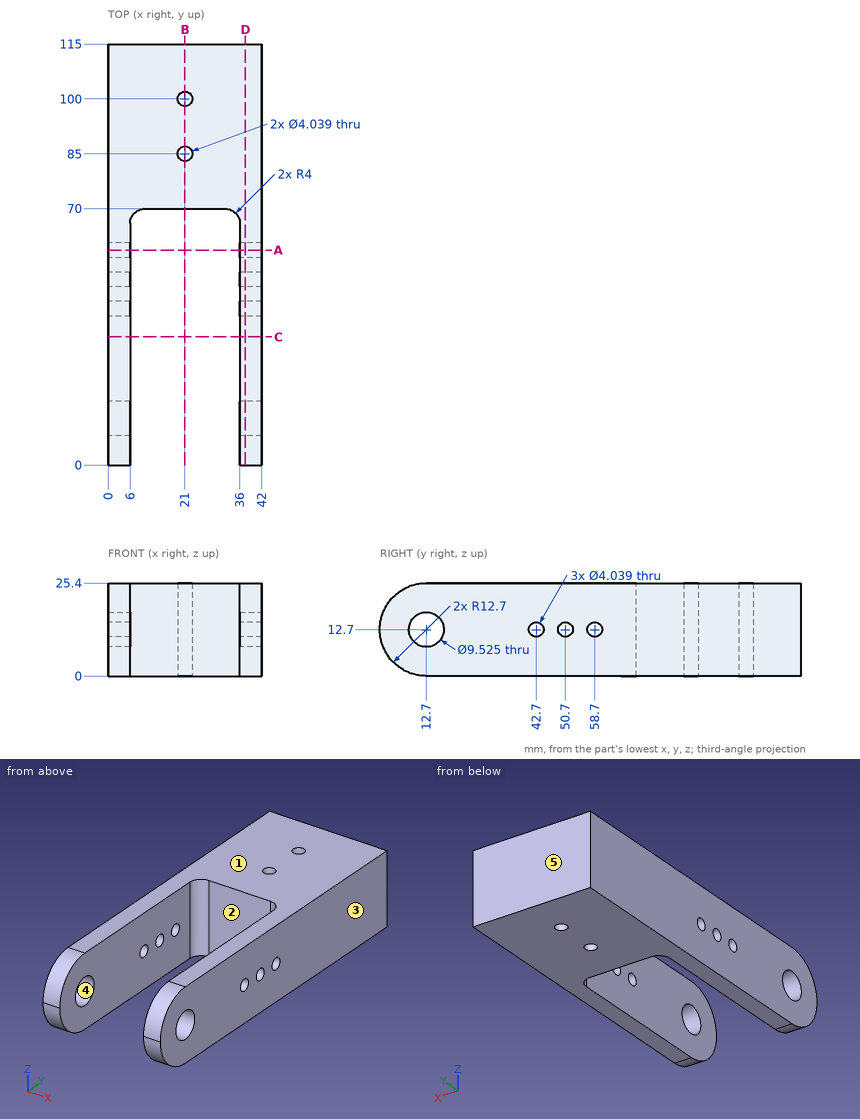
Could you check a few things on this drawing? It's one solid part, dimensions in mm from its lowest x, y, z. A direction names the side the tool comes from. Round coordinates to 2 decimals unless told otherwise and drop trailing zeros. Write each loop counter-clockwise with the first axis right and the second up, starting at its lowest first coordinate (ties: lowest second). Pieces come first, ordered by that corner, then holes.
Q1. If we section it at C-C on y = 35: Write out the boundary of the cut face in (x, z), plus the area to 3 significant figures.
Q2. Please list where these lines run through material, in increasing order: probe 1 along Y at (x, z) = (3.65, 12.7); probe 2 along Y at (x, z) = (21, 15.75); probe 3 along X at (y, z) = (35.5, 15.5).
Q3. If we section it at B-B on x = 21: Write out the boundary of the cut face in (y, z), plus the area to 3 significant figures.
Q4. If we section it at A-A on y = 58.7: Write out the boundary of the cut face in (x, z), plus the area to 3 significant figures.
Q5. If we mould it in two halves opening along Y, with no side actions, what happens to the marked faces 3, 4 and 5? For each: +Y half, -Y half, draft (parallel to the pull), parting line (faces both ways), or undercut.
Q6. Will these pins go through, and if not, where does the flat tip stop? P1, Ø4, axis at x = 9, z = 5, coming from the -Y side (1 decimal); P2, Ø11, axis at x = 16.5, z = 7.5, coming from the -Y side.
Q7. If we section it at D-D on x = 37.5: Give the number of separate pieces and of enclosed holes in the cut face, plus the area to 3 significant figures.
Q8. Which directions (+Z, -Z, +X, -X, +Y, -Y) give clear straight access to the entire face, cutting with the end or side of a thin tool? Please do the marked faces 1 and 2.
Answer below:
1. outline: (0, 0) - (6, 0) - (6, 25.4) - (0, 25.4) - close; (36, 0) - (42, 0) - (42, 25.4) - (36, 25.4) - close
1. area: 305 mm2
2. probe 1: y = 0 to 7.94, 17.46 to 40.68, 44.72 to 48.68, 52.72 to 56.68, 60.72 to 115
2. probe 2: y = 70 to 82.98, 87.02 to 97.98, 102.02 to 115
2. probe 3: x = 0 to 6, 36 to 42
3. outline: (70, 0) - (82.98, 0) - (82.98, 25.4) - (70, 25.4) - close; (87.02, 0) - (97.98, 0) - (97.98, 25.4) - (87.02, 25.4) - close; (102.02, 0) - (115, 0) - (115, 25.4) - (102.02, 25.4) - close
3. area: 938 mm2
4. outline: (0, 0) - (6, 0) - (6, 10.68) - (0, 10.68) - close; (0, 14.72) - (6, 14.72) - (6, 25.4) - (0, 25.4) - close; (36, 0) - (42, 0) - (42, 10.68) - (36, 10.68) - close; (36, 14.72) - (42, 14.72) - (42, 25.4) - (36, 25.4) - close
4. area: 256 mm2
5. face 3: draft
5. face 4: undercut
5. face 5: +Y half
6. P1: stops at y = 68.6
6. P2: stops at y = 70
7. separate pieces: 1
7. enclosed holes: 4
7. area: 2,740 mm2
8. face 1: +Z, +X, -X, +Y, -Y
8. face 2: +Z, -Z, -Y
